```python
from build123d import *

# Parameters (mm, degrees)
SKETCH1_R           = 42.5
SKETCH1_R_2         = 18.5
SKETCH1_R_3         = 1.75
BOSS_EXTRUDE1_DEPTH = 2.5
BOSS_EXTRUDE2_START = -14
SKETCH2_R           = 33.75
SKETCH2_R_2         = 18.5
BOSS_EXTRUDE2_DEPTH = 14
BOSS_EXTRUDE3_START = 15
SKETCH3_R           = 33.75
SKETCH3_R_2         = 30.5
BOSS_EXTRUDE3_DEPTH = 15


with BuildPart() as part:
    # Sketch1 → Boss-Extrude1 (new, symmetric)
    with BuildSketch(Plane(origin=(0, 0, 0), x_dir=(1, 0, 0), z_dir=(0, 1, 0))):
        with Locations(Location((0, 0, 0), (0, 0, 270))):
            Circle(SKETCH1_R)
        with Locations(Location((0, 0, 0), (0, 0, 270))):
            Circle(SKETCH1_R_2, mode=Mode.SUBTRACT)
        with Locations(Location((0, 37.5, 0), (0, 0, 270))):
            Circle(SKETCH1_R_3, mode=Mode.SUBTRACT)
        with Locations(Location((26.516504294, 26.516504294, 0), (0, 0, 270))):
            Circle(SKETCH1_R_3, mode=Mode.SUBTRACT)
        with Locations(Location((37.5, 0, 0), (0, 0, 270))):
            Circle(SKETCH1_R_3, mode=Mode.SUBTRACT)
        with Locations(Location((26.516504294, -26.516504294, 0), (0, 0, 270))):
            Circle(SKETCH1_R_3, mode=Mode.SUBTRACT)
        with Locations(Location((0, -37.5, 0), (0, 0, 270))):
            Circle(SKETCH1_R_3, mode=Mode.SUBTRACT)
        with Locations(Location((-26.516504294, -26.516504294, 0), (0, 0, 270))):
            Circle(SKETCH1_R_3, mode=Mode.SUBTRACT)
        with Locations(Location((-37.5, 0, 0), (0, 0, 270))):
            Circle(SKETCH1_R_3, mode=Mode.SUBTRACT)
        with Locations(Location((-26.516504294, 26.516504294, 0), (0, 0, 270))):
            Circle(SKETCH1_R_3, mode=Mode.SUBTRACT)
    extrude(amount=BOSS_EXTRUDE1_DEPTH, both=True)

    # Sketch2 → Boss-Extrude2 (add)
    with BuildSketch(Plane(origin=(0, -2.5, 0), x_dir=(1, 0, 0), z_dir=(0, 1, 0)).offset(BOSS_EXTRUDE2_START)):
        with Locations(Location((0, 0, 0), (0, 0, 270))):
            Circle(SKETCH2_R)
        with Locations(Location((0, 0, 0), (0, 0, 270))):
            Circle(SKETCH2_R_2, mode=Mode.SUBTRACT)
    extrude(amount=BOSS_EXTRUDE2_DEPTH)

    # Sketch3 → Boss-Extrude3 (add)
    with BuildSketch(Plane.XZ.offset(16.5).offset(BOSS_EXTRUDE3_START)):
        with Locations(Location((0, 0, 0), (0, 0, 90))):
            Circle(SKETCH3_R)
        with Locations(Location((0, 0, 0), (0, 0, 270))):
            Circle(SKETCH3_R_2, mode=Mode.SUBTRACT)
    extrude(amount=-BOSS_EXTRUDE3_DEPTH)


solid = part.part
```
Input: part model. Units: mm. Frame: model coordinates. A direction names the side the tool comes from. Give positions to 0.01 mm unless a question says otherwise; leave off trailing zeros. Order: outer loops, then holes, each group sorted by start corner. A loop starts at its lowest first (then second) coordinate and runs counter-clockwise, first axis right, second up. Notation, with made-up numbers: (49, 40.25) - (63, 40.25) arc R21 cw to (63, 72.25) - close; hole circle Ø10 at (23, 80). An arc over 180 degrees is marked (long way). Use a Markdown table: item, result.
(1) Pin query (flat end, axial travel): pin 1 (8 mm diameter, centred on y = -13, z = 19, fed in from -X); pin 2 (2 mm diameter, centred on y = -11, z = 12.5, fed in from -X); pin 3 (2 mm diameter, centred on x = -18, y = -11.5, fed in from +Z); pin 4 (3 mm diameter, centred on x = -26.52, z = 26.52, fed in from -Y). Return the tip coordinate at first contact, or that it passes through.
Computed values:
| item | result |
|---|---|
| pin 1 | stops at x = -30.23 |
| pin 2 | stops at x = -31.73 |
| pin 3 | stops at z = 29.16 |
| pin 4 | passes through |
(2) Section query B-B (z = 37.5). Output: boundary loops of the cut face in (x, y), then the cut area to 4 significant figures.
Computed values:
| item | result |
|---|---|
| outline | (-20, -2.5) - (-1.75, -2.5) - (-1.75, 2.5) - (-20, 2.5) - close; (1.75, -2.5) - (20, -2.5) - (20, 2.5) - (1.75, 2.5) - close |
| area | 182.5 mm2 |
(3) Draft query along X for faces 3 (the flat face through (30, -31.5, -8)), 4 (the cylindrical face through (35.79, -0.04, -0.38)), 5 (the cylindrical face through (29.942, -17.203, 15.574)). Return one class per face: released by +X, released by -X, zero draft, split by the parting line, or undercut.
Computed values:
| item | result |
|---|---|
| face 3 | zero draft |
| face 4 | undercut |
| face 5 | split by the parting line |
(4) Line query: line 1 (X direction, y = -1, z = 0); line 2 (X direction, y = -28, z = 1); line 3 (Y direction, x = 17, z = 10.5). Output: solid intervals per line, ascending. Write a range as from..to.
Computed values:
| item | result |
|---|---|
| line 1 | x = -42.5..-39.25, -35.75..-18.5, 18.5..35.75, 39.25..42.5 |
| line 2 | x = -33.74..-30.48, 30.48..33.74 |
| line 3 | y = -16.5..2.5 |
(5) Section query D-D (y = -6.5). Output: boundary loops of the cut face in (x, z).
Computed values:
| item | result |
|---|---|
| outline | circle Ø67.5 at (0, 0); hole circle Ø37 at (0, 0) |
(6) Section query C-C (x = 37.5). Output: boundary loops of the cut face in (y, z).
Computed values:
| item | result |
|---|---|
| outline | (-2.5, -20) - (2.5, -20) - (2.5, -1.75) - (-2.5, -1.75) - close; (-2.5, 1.75) - (2.5, 1.75) - (2.5, 20) - (-2.5, 20) - close |
(7) Section query A-A (x = 0). Output: boundary loops of the cut face in (y, z).
Computed values:
| item | result |
|---|---|
| outline | (-31.5, -33.75) - (-2.5, -33.75) - (-2.5, -35.75) - (2.5, -35.75) - (2.5, -18.5) - (-16.5, -18.5) - (-16.5, -30.5) - (-31.5, -30.5) - close; (-31.5, 30.5) - (-16.5, 30.5) - (-16.5, 18.5) - (2.5, 18.5) - (2.5, 35.75) - (-2.5, 35.75) - (-2.5, 33.75) - (-31.5, 33.75) - close; (-2.5, -42.5) - (2.5, -42.5) - (2.5, -39.25) - (-2.5, -39.25) - close; (-2.5, 39.25) - (2.5, 39.25) - (2.5, 42.5) - (-2.5, 42.5) - close |
(8) Access query for faces 1 (the cylindrical face through (-25.861, 0.035, -33.727)), 2 (the cylindrical face through (-29.775, -24.105, 6.612)). Directions: +Z, -Z, +X, -X, +Y, -Y. A direction counts if a zero-diameter tool reaches every point of the face in a straight line with its end or side. Return the directions, or none.
Computed values:
| item | result |
|---|---|
| face 1 | +Y, -Y |
| face 2 | -Y |
